Could you check a few things on this model? Use its own coordinates, in mm. Face numbers are marked on the shaded views. Give positions to 0.01 mm unless a question says otherwise; leave off trailing zeros. Write each loop counter-clockwise with the first axis right and the second up, starting at its lowest first coordinate (ties: lowest second). Pieces come first, ordered by that corner, then holes. Notation, with made-up numbers: (16.25, -17.5) - (20.25, -17.5) arc R23 ccw to (20.25, 19.5) - close; hole circle Ø2 at (2.25, 69.5). An arc over 180 degrees is marked (long way). Write item = value, one per line.
from build123d import *

# Parameters (mm, degrees)
SKETCH1_W           = 508
SKETCH1_H           = 508
BOSS_EXTRUDE1_DEPTH = 4
SKETCH3_W           = 406.4
SKETCH3_H           = 406.4
CUT_EXTRUDE1_DEPTH  = 4
SKETCH4_W           = 508
SKETCH4_H           = 508
BOSS_EXTRUDE2_DEPTH = 1
SKETCH5_W           = 10
SKETCH5_H           = 30
CUT_EXTRUDE2_DEPTH  = 5


with BuildPart() as part:
    # Sketch1 → Boss-Extrude1 (new body)
    with BuildSketch(Plane.XY):
        with Locations((-254, 254)):
            Rectangle(SKETCH1_W, SKETCH1_H)
    extrude(amount=BOSS_EXTRUDE1_DEPTH)

    # Sketch3 → Cut-Extrude1 (cut)
    with BuildSketch(Plane.XY.offset(4)):
        with Locations((-254, 254)):
            Rectangle(SKETCH3_W, SKETCH3_H)
    extrude(amount=-CUT_EXTRUDE1_DEPTH, mode=Mode.SUBTRACT)

    # Sketch4 → Boss-Extrude2 (add)
    with BuildSketch(Plane.XY.offset(4)):
        with Locations((-254, 254)):
            Rectangle(SKETCH4_W, SKETCH4_H)
    extrude(amount=BOSS_EXTRUDE2_DEPTH)

    # Sketch5 → Cut-Extrude2 (cut)
    with BuildSketch(Plane(origin=(0, 0, 0), x_dir=(-1, 0, 0), z_dir=(0, 0, -1))):
        with Locations((5, 493)):
            Rectangle(SKETCH5_W, SKETCH5_H)
        with Locations((503, 493)):
            Rectangle(SKETCH5_W, SKETCH5_H)
        with Locations((503, 15)):
            Rectangle(SKETCH5_W, SKETCH5_H)
        with Locations((5, 15)):
            Rectangle(SKETCH5_W, SKETCH5_H)
    extrude(amount=-CUT_EXTRUDE2_DEPTH, mode=Mode.SUBTRACT)


solid = part.part
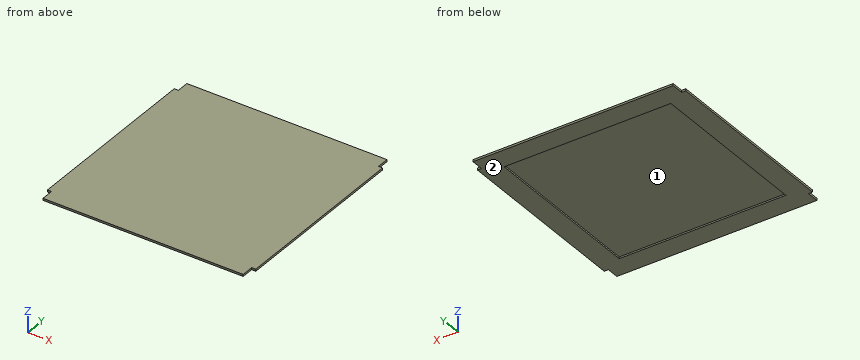
1. If we section it at C-C, the plane x = -109: Please give me the cut outline in (y, z), and give its area (3 significant figures).
Filled sheet:
outline = (0, 0) - (50.8, 0) - (50.8, 4) - (457.2, 4) - (457.2, 0) - (508, 0) - (508, 5) - (0, 5) - close
area = 914 mm2
2. If we section it at A-A, the plane z = 1.35: Please give me the cut outline in (x, y).
Filled sheet:
outline = (-508, 30) - (-498, 30) - (-498, 0) - (-10, 0) - (-10, 30) - (0, 30) - (0, 478) - (-10, 478) - (-10, 508) - (-498, 508) - (-498, 478) - (-508, 478) - close; hole (-457.2, 50.8) - (-50.8, 50.8) - (-50.8, 457.2) - (-457.2, 457.2) - close
3. Thinking about a two-plate mould opening in X: for the marked faces 1 and 2, which applies, pulls with the +X half, pulls with the -X half, needs draft (parallel to the pull), parting line crosses it, or undercut?
Filled sheet:
face_1 = undercut
face_2 = needs draft
4. I need wall thicknesses on line 1 (Y direction, x = -229.5, z = 1.8); line 2 (X direction, y = 91, z = 0.85); line 3 (Z direction, x = -403, y = 314.5). Which ranges of each line are inside material? Lowest first, please.
Filled sheet:
line_1 = 0 to 50.8, 457.2 to 508
line_2 = -508 to -457.2, -50.8 to 0
line_3 = 4 to 5
5. For pin 1 (1.5 mm diameter, centred on y = 9.5, z = 2, fed in from -X); pin 2 (1.5 mm diameter, centred on x = -502.5, z = 3, fed in from +Y); pin 3 (1.5 mm diameter, centred on x = -443.5, y = 407, fed in from -Z), each with a flat end and sliding along its axis, tell me the tip position at first contact or that it passes through.
Filled sheet:
pin_1 = -498
pin_2 = 478
pin_3 = 4
6. If we section it at B-B, the plane y = 71.5: Please give me the cut outline in (x, z).
Filled sheet:
outline = (-508, 0) - (-457.2, 0) - (-457.2, 4) - (-50.8, 4) - (-50.8, 0) - (0, 0) - (0, 5) - (-508, 5) - close
